Source: three-view drawing plus pictorial views. Frame: mm from the lowest corner of the part. A direction names the side the tool comes from. Give positions to 0.01 mm unless a question says otherwise; leave off trailing zeros. Order: outer loops, then holes, each group sorted by start corner. A loop starts at its lowest first (then second) coordinate and runs counter-clockwise, first axis right, second up.
1) Section C-C, the plane y = 28. Return loops of the section in (x, z), plus the area to 3 significant figures.
2) Material intervals for line 1 (Z direction, x = 17, y = 30.5); line 2 (X direction, y = 19, z = 1.25) (1 decimal); line 3 (Y direction, x = 7, z = 16.25) (1 decimal), sorted ascending.
3) Section A-A, the plane x = 14.5. Return loops of the section in (y, z).
4) Access query for the marked faces 5 and 6. Directions: +Z, -Z, +X, -X, +Y, -Y. A direction counts if a zero-diameter tool reaches every point of the face in a straight line with its end or side. Return the directions, or none.
5) Section D-D, the plane z = 15.5. Return loops of the section in (x, y).
6) Draft query along Y for the marked faces 1, 2, 3 and 4. Return one class per face: released by +Y, released by -Y, zero draft, split by the parting line, or undercut.
7) Section B-B, the plane y = 19. Return loops of the section in (x, z) (1 decimal).
8) First-contact query: P1, Ø2, axis at y = 5.5, z = 4.5, coming from the +X side; P2, Ø3, axis at x = 24.5, z = 6, coming from the -Y side; P3, Ø10, axis at x = 27, y = 21, coming from the -Z side. Flat tips, straight axial feed; report the tip coordinate or a pass-through.
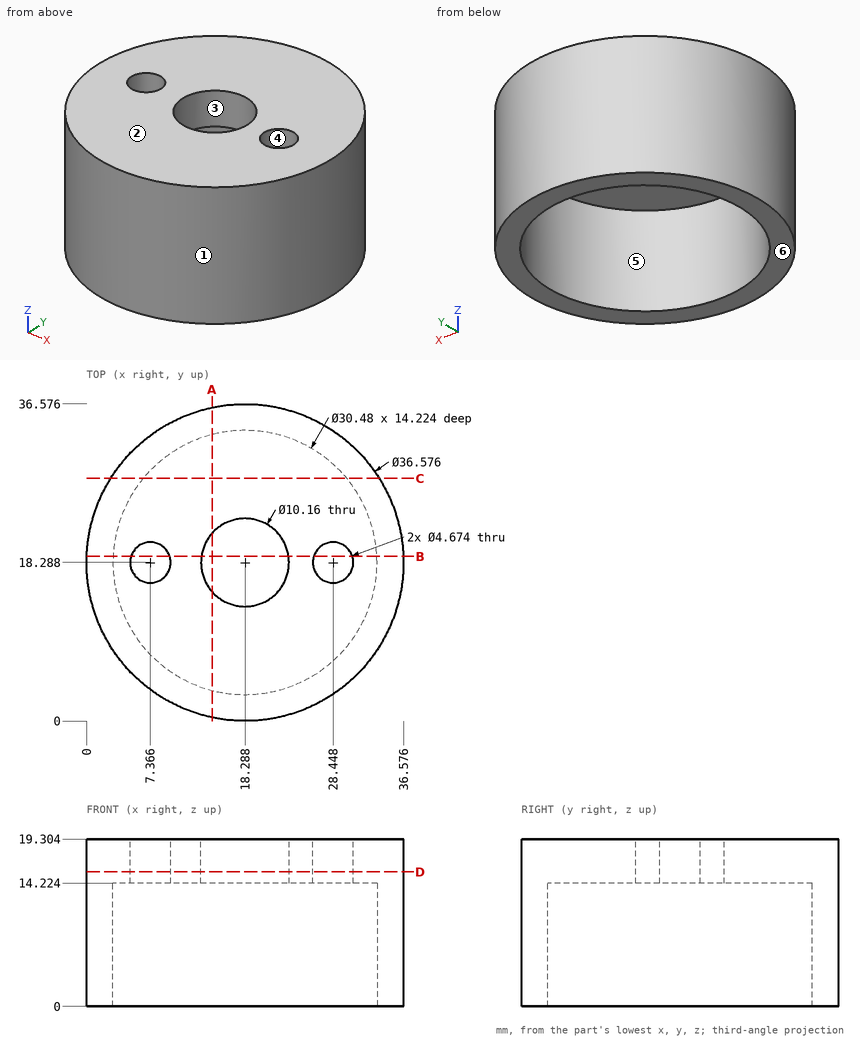
From the geometry:
1. outline: (2.79, 0) - (6.54, 0) - (6.54, 14.22) - (30.03, 14.22) - (30.03, 0) - (33.78, 0) - (33.78, 19.3) - (2.79, 19.3) - close
1. area: 264 mm2
2. line 1: z = 14.22 to 19.3
2. line 2: x = 0 to 3.1, 33.5 to 36.6
2. line 3: y = 3.9 to 16, 20.6 to 32.7
3. outline: (0.4, 0) - (3.53, 0) - (3.53, 14.22) - (14.9, 14.22) - (14.9, 19.3) - (0.4, 19.3) - close; (21.67, 14.22) - (33.05, 14.22) - (33.05, 0) - (36.18, 0) - (36.18, 19.3) - (21.67, 19.3) - close
4. face 5: -Z
4. face 6: -Z, +X, -X, +Y, -Y
5. outline: circle Ø36.58 at (18.29, 18.29); hole circle Ø4.67 at (7.37, 18.29); hole circle Ø10.16 at (18.29, 18.29); hole circle Ø4.67 at (28.45, 18.29)
6. face 1: split by the parting line
6. face 2: zero draft
6. face 3: undercut
6. face 4: undercut
7. outline: (0, 0) - (3.1, 0) - (3.1, 14.2) - (5.1, 14.2) - (5.1, 19.3) - (0, 19.3) - close; (9.6, 14.2) - (13.3, 14.2) - (13.3, 19.3) - (9.6, 19.3) - close; (23.3, 14.2) - (26.2, 14.2) - (26.2, 19.3) - (23.3, 19.3) - close; (30.7, 14.2) - (33.5, 14.2) - (33.5, 0) - (36.6, 0) - (36.6, 19.3) - (30.7, 19.3) - close
8. P1: stops at x = 32.27
8. P2: stops at y = 0.62
8. P3: stops at z = 14.22
